from build123d import *

# Parameters (mm, degrees)
F0_W     = 134.62
F0_H     = 134.62
F0_R     = 2.286
F0_R_2   = 51.435
F4_DEPTH = 6.35
F2_W     = 134.62
F2_H     = 134.62
F2_R     = 2.286
F2_R_2   = 49.53
F7_DEPTH = 3.81
F6_W     = 134.62
F6_H     = 134.62
F6_R     = 2.286
F6_R_2   = 46.355
F8_DEPTH = 2.54


# Not quite as in the source:
# - the program builds the solid bodies; features that only make, move or delete a surface that nothing else refers to are left out


with BuildPart() as f4:
    # F0 (on Top) → F4 (new body)
    with BuildSketch(Plane.XY):
        Rectangle(F0_W, F0_H)
        with Locations((-43.1052293811, -43.1052293811)):
            Circle(F0_R, mode=Mode.SUBTRACT)
        with Locations((43.2547706189, -43.5552815736)):
            Circle(F0_R, mode=Mode.SUBTRACT)
        with Locations((-42.9551675437, 43.2547706189)):
            Circle(F0_R, mode=Mode.SUBTRACT)
        Circle(F0_R_2, mode=Mode.SUBTRACT)
        with Locations((43.4036597586, 42.8047184264)):
            Circle(F0_R, mode=Mode.SUBTRACT)
    extrude(amount=-F4_DEPTH)

    # F2 (on offset) → F7 (join)
    with BuildSketch(Plane.XY.offset(-2.54)):
        Rectangle(F2_W, F2_H)
        with Locations((-43.1052293811, -43.1052293811)):
            Circle(F2_R, mode=Mode.SUBTRACT)
        with Locations((43.2547706189, -43.5552815736)):
            Circle(F2_R, mode=Mode.SUBTRACT)
        with Locations((-42.9551675437, 43.2547706189)):
            Circle(F2_R, mode=Mode.SUBTRACT)
        Circle(F2_R_2, mode=Mode.SUBTRACT)
        with Locations((43.4036597586, 42.8047184264)):
            Circle(F2_R, mode=Mode.SUBTRACT)
    extrude(amount=-F7_DEPTH)

    # F6 (on offset) → F8 (join)
    with BuildSketch(Plane.XY.offset(-3.81)):
        Rectangle(F6_W, F6_H)
        with Locations((-43.1052293811, -43.1052293811)):
            Circle(F6_R, mode=Mode.SUBTRACT)
        with Locations((43.2547706189, -43.5552815736)):
            Circle(F6_R, mode=Mode.SUBTRACT)
        with Locations((-42.9551675437, 43.2547706189)):
            Circle(F6_R, mode=Mode.SUBTRACT)
        Circle(F6_R_2, mode=Mode.SUBTRACT)
        with Locations((43.4036597586, 42.8047184264)):
            Circle(F6_R, mode=Mode.SUBTRACT)
    extrude(amount=-F8_DEPTH)


solid = f4.part
Can you work these out from the model? Positions are in its coordinate system, mm. A direction names the side the tool comes from. Round coordinates to 2 decimals unless told otherwise and drop trailing zeros. Loops run counter-clockwise (first coordinate to the right, second up) from the corner with the lowest first, then second, coordinate; pieces in that order, holes last. Notation, with made-up numbers: (80, 63.5) - (97, 63.5) arc R12 ccw to (97, 68.5) - close; hole circle Ø5 at (-18.5, 7.5). An arc over 180 degrees is marked (long way). Use CSV: the item, a comma, the result in double quotes. Start each with the question number.
1) For pin 1 Ø8 at (x, y) = (18, -35) entering from -Z, with a flat end and sliding along its axis, tell me the tip position at first contact or that it passes through.
2) If we section it at C-C on z = -5.25: Write out the boundary of the cut face in (x, y) (3 decimals).
3) Please list where these lines run through material, in increasing order: probe 1 along Y at (x, z) = (0, -3); probe 2 along Y at (x, z) = (-45, -3.5); probe 3 along X at (y, z) = (-45, -1.5). Write a range as [from, to].
4) For faces 4 (the flat face through (-67.31, -1, -3)), 5 (the cylindrical face through (-40.817, -31.297, -1.252)), which set-ups out of +Z, -Z, +X, -X, +Y, -Y let a thin tool reach every point of the face, with its end or its side?
5) We'd pull the mould along X, two halves only. Please class faces 1 (the flat face through (-1, -67.31, -3)), 2 (the flat face through (67.31, -1, -3)), 3 (the cylindrical face through (45.435, -42.869, -3.131)): released by +X, released by -X, zero draft, split by the parting line, or undercut.
6) If we section it at A-A on y = 0: Write out the boundary of the cut face in (x, z) (3 decimals), plus the area to 3 significant figures.
Geometry results:
1,pin 1,"passes through"
2,outline,"(-67.31, -67.31) - (67.31, -67.31) - (67.31, 67.31) - (-67.31, 67.31) - close; hole circle Ø92.71 at (0, 0); hole circle Ø4.572 at (-43.105, -43.105); hole circle Ø4.572 at (-42.955, 43.255); hole circle Ø4.572 at (43.255, -43.555); hole circle Ø4.572 at (43.404, 42.805)"
3,probe 1,"y = [-67.31, -49.53], [49.53, 67.31]"
3,probe 2,"y = [-67.31, -44.38], [-41.83, -20.69], [20.69, 42.23], [44.28, 67.31]"
3,probe 3,"x = [-67.31, -44.38], [-41.83, -24.91], [24.91, 41.48], [45.03, 67.31]"
4,face 4,"+Z, -Z, -X, +Y, -Y"
4,face 5,"+Z"
5,face 1,"zero draft"
5,face 2,"released by +X"
5,face 3,"undercut"
6,outline,"(-67.31, -6.35) - (-46.355, -6.35) - (-46.355, -3.81) - (-49.53, -3.81) - (-49.53, -2.54) - (-51.435, -2.54) - (-51.435, 0) - (-67.31, 0) - close; (46.355, -6.35) - (67.31, -6.35) - (67.31, 0) - (51.435, 0) - (51.435, -2.54) - (49.53, -2.54) - (49.53, -3.81) - (46.355, -3.81) - close"
6,area,"232 mm2"
